Read the model definition and answer for the solid it produces. Units are mm, in the model's axes. Coordinates: 2 decimals unless noted, no trailing zeros. Loops run counter-clockwise (first coordinate to the right, second up) from the corner with the lowest first, then second, coordinate; pieces in that order, holes last. Notation, with made-up numbers: (77, -3) - (127, -3) arc R19 cw to (127, 25) - close; hole circle Ø4 at (-4, 0.5). An arc over 180 degrees is marked (long way). One line per item, written item: value. Start each with the question number.
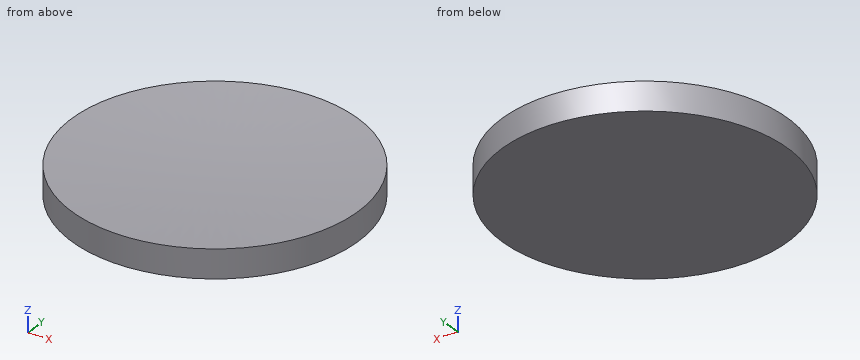
from build123d import *

# Parameters (mm, degrees)
CYLINDER001_R     = 50
CYLINDER001_DEPTH = 10


with BuildPart() as sphere001:
    # Sphere001 → Sphere001 (revolve)
    with BuildSketch(Plane(origin=(0, 0, 607.913037), x_dir=(1, 0, 0), z_dir=(0, -1, 0))):
        with BuildLine():
            ThreePointArc((0, -600), (600, 0), (0, 600))
            Line((0, 600), (0, -600))
        make_face()
    revolve(axis=Axis((0, 0, 607.913037), (0, 0, 1)))


with BuildPart() as concavemirror:
    # Cylinder001 → Cylinder001 (new body)
    with BuildSketch(Plane.XY):
        Circle(CYLINDER001_R)
    extrude(amount=CYLINDER001_DEPTH)

    # Cut001: cut Sphere001
    add(sphere001.part, mode=Mode.SUBTRACT)


solid = concavemirror.part
1) Flat-ended cylindrical pins translate along their axes: P1, Ø4, axis at x = 38, z = 7.5, coming from the +Y side; P2, Ø1, axis at x = -16, y = -30, coming from the +Z side; P3, Ø3, axis at x = 33, z = 4.5, coming from the -Y side. Find the tip coordinate at first contact, or state that the pin passes through.
2) Section C-C, the plane z = 2 is taken. Determine the outline of the cut face in (x, y), and give its area (3 significant figures).
3) Section A-A, the plane x = 0 is taken. Determine the outline of the cut face in (y, z), and give its area (3 significant figures).
4) Straight lines are drawn through the part: L1, parallel to Z at x = 19.5, y = 37; L2, parallel to Z at x = -6, y = -20; L3, parallel to X at y = -35.5, z = 4.5. For each, find the intervals that lie inside material, in ascending order.
Answer below:
1. P1: y = 34.7
1. P2: z = 8.91
1. P3: y = -38.83
2. outline: circle Ø100 at (0, 0)
2. area: 7,850 mm2
3. outline: (-50, 0) - (50, 0) - (50, 10) arc R600 cw to (-50, 10) - close
3. area: 861 mm2
4. L1: 0 to 9.37
4. L2: 0 to 8.28
4. L3: -35.21 to 35.21
